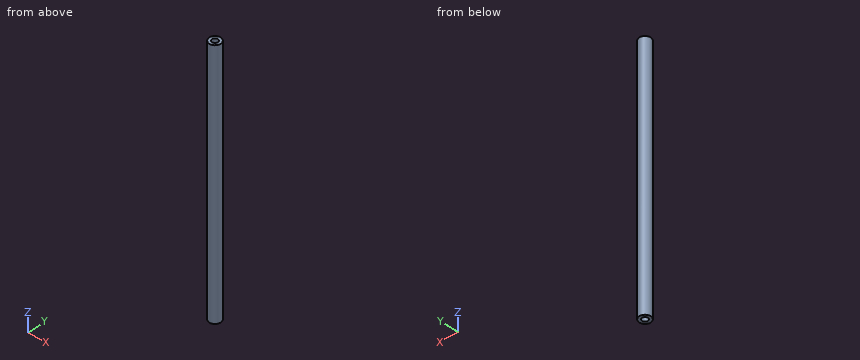
Autodesk Inventor part; units mm, degrees
ref_plane "YZ Plane" through (0, 0, 0) normal (1, 0, 0) x (0, 1, 0)
ref_plane "XZ Plane" through (0, 0, 0) normal (0, 1, 0) x (-1, 0, 0)
ref_plane "XY Plane" through (0, 0, 0) normal (0, 0, 1) x (1, 0, 0)
sketch "スケッチ1" plane through (0, 0, 0) normal (0, 0, 1) x (1, 0, 0)
  circle A0 centre (0, 0) radius 2
  circle A1 centre (0, 0) radius 4
  dimension "d0" = 4
  dimension "d1" = 8
extrude "押し出し1" add sketch "スケッチ1" along normal mid plane 177 contours A0 | A1
sketch "スケッチ3" plane through (0, 0, 88.5) normal (0, 0, 1) x (1, 0, 0)
  circle A0 centre (0, 0) radius 2
  dimension "d5" = 4
extrude "押し出し2" cut sketch "スケッチ3" against normal blind 10
sketch "スケッチ4" plane through (0, 0, -88.5) normal (0, 0, -1) x (-1, 0, 0)
  circle A0 centre (0, 0) radius 2
  dimension "d8" = 4
extrude "押し出し3" cut sketch "スケッチ4" against normal blind 10
properties part number "シャフト177mm" material "アルミニウム 7075"
Model file for the job. Use its own axes, mm. Round coordinates to 2 decimals unless told otherwise and drop trailing zeros. Write each loop counter-clockwise with the first axis right and the second up, starting at its lowest first coordinate (ties: lowest second). Pieces come first, ordered by that corner, then holes. Notation, with made-up numbers: (68, 6) - (76, 6) arc R20 ccw to (76, 28) - close; hole circle Ø6 at (7.25, 25.5). An arc over 180 degrees is marked (long way). Use CSV: the item, a comma, the result in double quotes. Start each with the question number.
Item 1: Band-saw the part on A-A (y = 0). Write the cut outline in (x, z), and give its area (3 significant figures).
Item 2: Band-saw the part on C-C (z = 46.5). Write the cut outline in (x, y), and give its area (3 significant figures).
Item 3: Pin check, flat tips, straight feed: P1, Ø1, axis at x = 1.5, z = -25, coming from the +Y side; P2, Ø1.5, axis at x = 1, y = 0, coming from the -Z side; P3, Ø2, axis at x = 2.5, z = -57.5, coming from the +Y side. Stop position of each tip, or through.
Item 4: Drill centre lines: L1, parallel to Y at x = 0, z = 83.75; L2, parallel to Y at x = 0.25, z = -38.5. Where is each one in solid material? Low to high. Write a range as [from, to].
Checked values:
1,outline,"(-4, -88.5) - (-2, -88.5) - (-2, -78.5) - (2, -78.5) - (2, -88.5) - (4, -88.5) - (4, 88.5) - (2, 88.5) - (2, 78.5) - (-2, 78.5) - (-2, 88.5) - (-4, 88.5) - close"
1,area,"1,340 mm²"
2,outline,"circle Ø8 at (0, 0)"
2,area,"50.3 mm²"
3,P1,"stops at y = 3.87"
3,P2,"stops at z = -78.5"
3,P3,"stops at y = 3.71"
4,L1,"y = [-4, -2], [2, 4]"
4,L2,"y = [-3.99, 3.99]"
